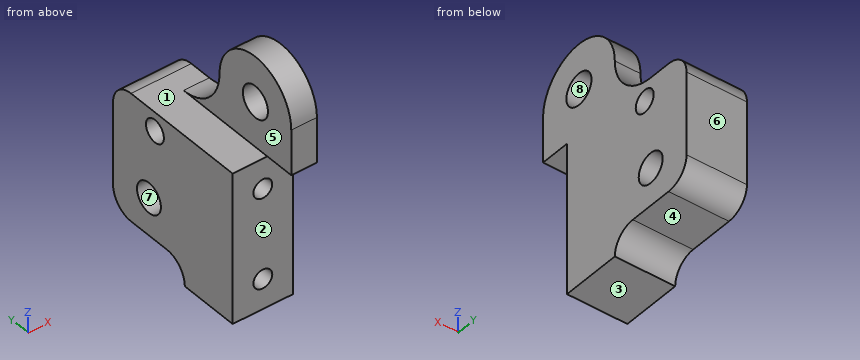
```python
from build123d import *

# Parameters (mm, degrees)
SKETCH1_R                       = 1.5
SKETCH1_R_2                     = 2
BOSS_EXTRUDE1_DEPTH             = 8
FILLET1_R                       = 3
FILLET2_R                       = 6
TAP_DRILL_FOR_M5X0_8_TAP1_D     = 4.2
TAP_DRILL_FOR_M3X0_5_TAP1_D     = 2.5
TAP_DRILL_FOR_M3X0_5_TAP1_DEPTH = 6
TAP_DRILL_FOR_M3X0_5_TAP1_TIP   = 0.751075774
CUT_EXTRUDE1_REACH              = 38.277
SKETCH7_W                       = 4.6
SKETCH7_H                       = 12


with BuildPart() as part:
    # Sketch1 → Boss-Extrude1 (new body)
    with BuildSketch(Plane(origin=(0, 0, 0), x_dir=(0, 0, -1), z_dir=(1, 0, 0))):
        with BuildLine():
            Line((6, 0), (0, 0))
            ThreePointArc((0, 0), (-6, 6), (0, 12))
            Line((0, 12), (6, 12))
            Line((6, 12), (6, 24))
            Line((6, 24), (23, 24))
            Line((23, 24), (23, 12))
            Line((23, 12), (26, 12))
            Line((26, 12), (26, 4))
            Line((26, 4), (6, 4))
            Line((6, 4), (6, 0))
        make_face()
        with Locations((8.5, 17)):
            Circle(SKETCH1_R, mode=Mode.SUBTRACT)
        with Locations((18, 18)):
            Circle(SKETCH1_R_2, mode=Mode.SUBTRACT)
    extrude(amount=BOSS_EXTRUDE1_DEPTH)

    # Fillet1
    fillet1_edges = [part.edges().sort_by_distance(p)[0] for p in [
        (4, 12, -23),
        (4, 24, -6),
        (4, 24, -23),
    ]]
    fillet(fillet1_edges, radius=FILLET1_R - 0.0001)  # a hair under: the kernel refuses the full size

    # Fillet2
    fillet2_edges = [part.edges().sort_by_distance(p)[0] for p in [
        (4, 12, -6),
    ]]
    fillet(fillet2_edges, radius=FILLET2_R - 0.0001)  # a hair under: the kernel refuses the full size

    # Tap Drill for M5x0.8 Tap1 (through all)
    with Locations(Plane(origin=(8, 0, 0), x_dir=(0, 0, -1), z_dir=(1, 0, 0))):
        with Locations((0, 6)):
            Hole(TAP_DRILL_FOR_M5X0_8_TAP1_D / 2)

    # Tap Drill for M3x0.5 Tap1
    with Locations(Plane(origin=(0, 4, 0), x_dir=(-1, 0, 0), z_dir=(0, -1, 0))):
        with Locations((-4, 10), (-4, 22)):
            Hole(TAP_DRILL_FOR_M3X0_5_TAP1_D / 2, depth=TAP_DRILL_FOR_M3X0_5_TAP1_DEPTH)
            with Locations((0, 0, -(TAP_DRILL_FOR_M3X0_5_TAP1_DEPTH + TAP_DRILL_FOR_M3X0_5_TAP1_TIP / 2))):  # 118° drill point
                Cone(0, TAP_DRILL_FOR_M3X0_5_TAP1_D / 2, TAP_DRILL_FOR_M3X0_5_TAP1_TIP, mode=Mode.SUBTRACT)

    # Sketch7 → Cut-Extrude1 (cut, up to next)
    with BuildSketch(Plane.XZ, mode=Mode.PRIVATE) as cut_extrude1_sk1:
        with Locations((2.3, 0)):
            Rectangle(SKETCH7_W, SKETCH7_H)
    cut_extrude1_tool1 = extrude(cut_extrude1_sk1.sketch, amount=-CUT_EXTRUDE1_REACH, mode=Mode.PRIVATE) & part.part
    add(cut_extrude1_tool1.solids().sort_by_distance((2.3, 0, 0))[0], mode=Mode.SUBTRACT)


solid = part.part
```
Verification items for the finished model (mm, model axes). Face numbers are marked on the shaded views. A direction names the side the tool comes from. Coordinates: 2 decimals unless noted, no trailing zeros. Loops run counter-clockwise (first coordinate to the right, second up) from the corner with the lowest first, then second, coordinate; pieces in that order, holes last. Notation, with made-up numbers: (21.25, -40) -> (78.25, -40) arc R7 cw to (78.25, -27) -> close; hole circle Ø5 at (-24, -31.75). An arc over 180 degrees is marked (long way). Put each result on its own line as item: value.
1. Section check B-B, the plane y = 17. Record the boundary of the cut face in (x, z).
Result set:
outline: (0, -23) -> (8, -23) -> (8, -19.73) -> (0, -19.73) -> close; (0, -16.27) -> (8, -16.27) -> (8, -10) -> (0, -10) -> close; (0, -7) -> (8, -7) -> (8, -5.92) -> (4.6, -5.92) -> (4.6, -6) -> (0, -6) -> close
2. Gauge pin test, flat ends, axial feed: P1, Ø13, axis at y = 13, z = 1, coming from the -X side; P2, Ø3, axis at x = 3, z = -22.5, coming from the +Y side; P3, Ø4, axis at x = 4.5, y = 15, coming from the +Z side; P4, Ø1, axis at y = 17, z = -17, coming from the -X side. Record the tip position at first contact, or that the pin passes through.
Result set:
P1: stops at x = 4.6
P2: stops at y = 23.83
P3: stops at z = -3.32
P4: passes through
3. Thickness scan on line 1 (Z direction, x = 4, y = 6.85); line 2 (Y direction, x = 5.9, z = 0); line 3 (X direction, y = 5.4, z = -22). Record the ranges inside material, lowest first.
Result set:
line 1: z = -26 to -23.25, -20.75 to -11.25, -8.75 to -6
line 2: y = 0 to 3.9, 8.1 to 12
line 3: x = 0 to 2.75, 5.25 to 8
4. Mould release check, pull along Y, two halves, no side actions. Record for the marked faces 5, 6, 7 and 8: pulls with the +Y half, pulls with the -Y half, needs draft (parallel to the pull), parting line crosses it, or undercut.
Result set:
face 5: needs draft
face 6: pulls with the +Y half
face 7: undercut
face 8: undercut
5. Section check D-D, the plane z = -13. Record the boundary of the cut face in (x, y).
Result set:
outline: (0, 4) -> (8, 4) -> (8, 24) -> (0, 24) -> close
6. Section check C-C, the plane x = 0.5. Give the number of separate pieces and of enclosed holes in the cut face, then the cut area to 3 significant figures.
Result set:
separate pieces: 1
enclosed holes: 2
area: 342 mm^2
7. Section check A-A, the plane z = -16.5. Record the boundary of the cut face in (x, y).
Result set:
outline: (0, 4) -> (8, 4) -> (8, 16.68) -> (0, 16.68) -> close; (0, 19.32) -> (8, 19.32) -> (8, 24) -> (0, 24) -> close
8. Tool access check on the marked faces 1, 2, 3 and 4. Record the directions out of +Z, -Z, +X, -X, +Y, -Y that give a thin tool (end or side, any length) a straight path to the whole face; none if there is none.
Result set:
face 1: +Z, -X, +Y
face 2: -Z, +X, -X, -Y
face 3: -Z, +X, -X, +Y, -Y
face 4: -Z, +X, -X, +Y
